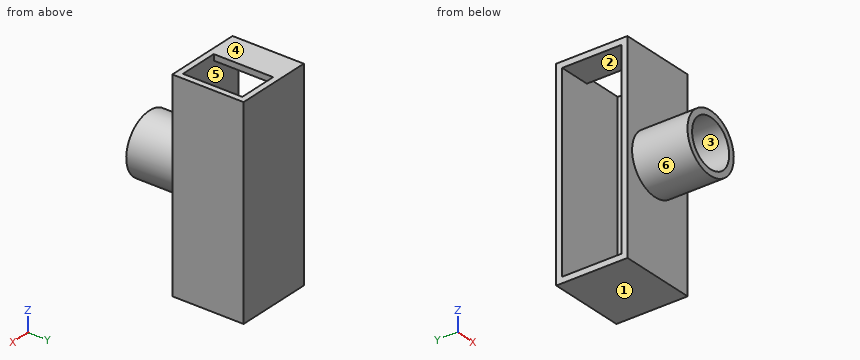
```python
from build123d import *

# Parameters (mm, degrees)
SKETCH_1_R          = 6
EXTRUDE_1_DEPTH     = 1.5
SKETCH_2_R          = 6
EXTRUDE_2_DEPTH     = 14
SKETCH_3_W          = 18
SKETCH_3_H          = 48
EXTRUDE_3_DEPTH     = 15
SHELL_3_T           = 1.5
SKETCH_4_W          = 10
SKETCH_4_H          = 15
CUT_EXTRUDE_1_DEPTH = 15


with BuildPart() as part:
    # 草图1 → 凸台-拉伸1 (new body)
    with BuildSketch(Plane(origin=(0, 0, 0), x_dir=(1, 0, 0), z_dir=(0, 1, 0))):
        with Locations(Location((0, 0, 0), (0, 0, 270))):
            Circle(SKETCH_1_R)
    extrude(amount=EXTRUDE_1_DEPTH)

    # 草图2 → 凸台-拉伸2 (add)
    with BuildSketch(Plane(origin=(0, 1.5, 0), x_dir=(1, 0, 0), z_dir=(0, 1, 0))):
        with Locations(Location((0, 0, 0), (0, 0, 270))):
            Circle(SKETCH_2_R)
    extrude(amount=EXTRUDE_2_DEPTH)

    # 草图3 → 凸台-拉伸3 (add)
    with BuildSketch(Plane(origin=(0, 15.5, 0), x_dir=(1, 0, 0), z_dir=(0, 1, 0))):
        Rectangle(SKETCH_3_W, SKETCH_3_H)
    extrude(amount=EXTRUDE_3_DEPTH)

    # 抽壳3
    shell_3_openings = [part.faces().sort_by_distance(p)[0] for p in [
        (-9, 23, 0),
        (0, 0, 0),
    ]]
    offset(amount=SHELL_3_T, openings=shell_3_openings, kind=Kind.INTERSECTION)

    # 草图4 → 切除-拉伸1 (cut)
    with BuildSketch(Plane(origin=(0, 0, 24), x_dir=(-1, 0, 0), z_dir=(0, 0, -1))):
        with Locations((-4, 23)):
            Rectangle(SKETCH_4_W, SKETCH_4_H)
    extrude(amount=-CUT_EXTRUDE_1_DEPTH, mode=Mode.SUBTRACT)


solid = part.part
```
The model under review builds one solid part; all positions refer to its coordinate system, in mm. Face numbers are marked on the shaded views. A direction names the side the tool comes from. Round coordinates to 2 decimals unless told otherwise and drop trailing zeros. Write each loop counter-clockwise with the first axis right and the second up, starting at its lowest first coordinate (ties: lowest second). Pieces come first, ordered by that corner, then holes. Notation, with made-up numbers: (39, 63.5) - (44, 63.5) arc R17 ccw to (44, 76.5) - close; hole circle Ø6 at (32.5, 6). An arc over 180 degrees is marked (long way). Answer as CSV lines item,"result". Start each with the question number.
(1) For pin 1 Ø4.5 at (y, z) = (22, 9) entering from -X; pin 2 Ø5.5 at (x, z) = (-1, 3.5) entering from -Y; pin 3 Ø1.5 at (x, z) = (4.5, -10) entering from -Y; pin 4 Ø1 at (x, z) = (-3, 0) entering from -Y, all flat-tipped, find the tip position at first contact; note any pin that passes through.
(2) Draft analysis for pull direction Z (two halves, no side actions). For the marked faces 4, 5 and 6, state which applies: pulls with the +Z half, pulls with the -Z half, needs draft (parallel to the pull), parting line crosses it, or undercut.
(3) We need section B-B on z = 0. State the section outline as (x, y) points.
(4) We need section C-C on y = 27. State the section outline as (x, z) points.
(5) We need section D-D on z = 21. State the section outline as (x, y) points, plus the area to 3 significant figures.
(6) To check wall thickness, follow line 1 (Y direction, x = 8.75, z = 20.5); line 2 (Y direction, x = 0, z = -6.5); line 3 (X direction, y = 11, z = 0). State the ranges of each line that lie inside material, in increasing order.
(7) We need section A-A on x = 0. State the section outline as (y, z) points.
(8) For the marked faces 1, 2 and 3, list the 3-axis set-ups (+Z, -Z, +X, -X, +Y, -Y) from which the entire face can be reached by the end or side of a thin tool; tool diameter is ignored.
Worked answers:
1,pin 1,"x = 9"
1,pin 2,"y = 0"
1,pin 3,"y = 14"
1,pin 4,"y = 30.5"
2,face 4,"pulls with the +Z half"
2,face 5,"undercut"
2,face 6,"parting line crosses it"
3,outline,"(-9, 14) - (-7.5, 14) - (-7.5, 0) - (-6, 0) - (-6, 15.5) - (-9, 15.5) - close; (-9, 30.5) - (9, 30.5) - (9, 15.5) - (6, 15.5) - (6, 0) - (7.5, 0) - (7.5, 14) - (10.5, 14) - (10.5, 32) - (-9, 32) - close"
4,outline,"(-9, -25.5) - (10.5, -25.5) - (10.5, 25.5) - (9, 25.5) - (9, -24) - (-9, -24) - close; (-9, 24) - (-1, 24) - (-1, 25.5) - (-9, 25.5) - close"
5,outline,"(-9, 14) - (10.5, 14) - (10.5, 32) - (-9, 32) - (-9, 30.5) - (9, 30.5) - (9, 15.5) - (-9, 15.5) - close"
5,area,"81.0 mm²"
6,line 1,"14 to 15.5, 30.5 to 32"
6,line 2,"0 to 15.5, 30.5 to 32"
6,line 3,"-7.5 to -6, 6 to 7.5"
7,outline,"(0, -7.5) - (14, -7.5) - (14, -25.5) - (32, -25.5) - (32, 25.5) - (30.5, 25.5) - (30.5, -24) - (15.5, -24) - (15.5, -6) - (0, -6) - close; (0, 6) - (15.5, 6) - (15.5, 25.5) - (14, 25.5) - (14, 7.5) - (0, 7.5) - close"
8,face 1,"-Z, +X, -X, +Y, -Y"
8,face 2,"-X"
8,face 3,"-Y"
